Source: CAD feature listing. Evaluate the final solid. Frame: model axes, mm. A direction names the side the tool comes from. Coordinates: 2 decimals unless noted, no trailing zeros. Write each loop counter-clockwise with the first axis right and the second up, starting at its lowest first coordinate (ties: lowest second). Pieces come first, ordered by that corner, then holes. Notation, with made-up numbers: (22, 0.25) - (45, 0.25) arc R21 cw to (45, 16.25) - close; hole circle Ø5 at (50.25, 53). An arc over 180 degrees is marked (long way). One line per question, with ' | ' between items. Start each with the question number.
Q1. Draft query along Z for faces 1 (the face through (-4, 0, -482.6)), 2 (the face through (111, 0, 185.737)), 3 (the face through (136.525, 0, 405)). Return one class per face: +Z half, -Z half, draft (parallel to the pull), parting line (faces both ways), or undercut.
Q2. Line query: line 1 (Z direction, x = -250.5, y = 5.25); line 2 (X direction, y = 4.5, z = -330.2) (3 decimals); line 3 (X direction, y = -0.25, z = 275) (3 decimals). Output: solid intervals per line, ascending.
Q3. Contact query for flat-ended pins moving along their axis: P1, Ø4, axis at y = 1.5, z = 157, coming from the -X side (3 decimals); P2, Ø7.5, axis at x = 103.5, y = -1, coming from the +Z side. Output: stop coordinate, or through.
Q4. Cut plane A-A, the plane x = 116.5. Give the number of separate pieces and of enclosed holes in the cut face, plus the area to 3 significant figures.
Q5. Access query for faces 4 (the face through (-239, 0, 249.238)), 5 (the face through (111, 0, 58.738)), 6 (the face through (214, 0, 482.6)). Directions: +Z, -Z, +X, -X, +Y, -Y. A direction counts if a zero-diameter tool reaches every point of the face in a straight line with its end or side. Return the directions, or none.
Q6. Cut plane B-B, the plane z = -134.5. Return loops of the section in (x, y) (3 decimals), plus the area to 3 significant figures.
```python
from build123d import *

# Parameters (mm, degrees)
F1_DEPTH = 12.7
F2_R     = 6.35
F3_DEPTH = 25.4
F4_R     = 9.525
F5_DEPTH = 25.4
F6_W     = 50.8
F6_H     = 12.7
F7_DEPTH = 25.4


with BuildPart() as f1:
    # F0 (on Front) → F1 (new body, symmetric)
    with BuildSketch(Plane.XZ):
        Polygon((-288.925, -406.4), (-288.925, -482.6), (288.925, -482.6), (288.925, 482.6), (136.525, 482.6), (136.525, 325.4375), (-288.925, 325.4375), (-288.925, 249.2375), (-187.325, 249.2375), (-187.325, -406.4), align=None)
    extrude(amount=F1_DEPTH, both=True)

    # F2 (on face) → F3 (cut)
    with BuildSketch(Plane.XZ.offset(12.7)):
        with Locations((231.775, -330.2)):
            Circle(F2_R)
    extrude(amount=-F3_DEPTH, mode=Mode.SUBTRACT)

    # F4 (on face) → F5 (cut)
    with BuildSketch(Plane.XZ.offset(12.7)):
        with Locations((34.759605, -194.841525)):
            Circle(F4_R)
    extrude(amount=-F5_DEPTH, mode=Mode.SUBTRACT)

    # F6 (on face) → F7 (cut)
    with BuildSketch(Plane.XZ.offset(12.7)):
        with Locations((111.125, 306.3875)):
            Rectangle(F6_W, F6_H)
        with Locations((111.125, 280.9875)):
            Rectangle(F6_W, F6_H)
        with Locations((111.125, 255.5875)):
            Rectangle(F6_W, F6_H)
        with Locations((111.125, 230.1875)):
            Rectangle(F6_W, F6_H)
        with Locations((111.125, 204.7875)):
            Rectangle(F6_W, F6_H)
        with Locations((111.125, 179.3875)):
            Rectangle(F6_W, F6_H)
        with Locations((111.125, 153.9875)):
            Rectangle(F6_W, F6_H)
        with Locations((111.125, 128.5875)):
            Rectangle(F6_W, F6_H)
        with Locations((111.125, 103.1875)):
            Rectangle(F6_W, F6_H)
        with Locations((111.125, 77.7875)):
            Rectangle(F6_W, F6_H)
        with Locations((111.125, 52.3875)):
            Rectangle(F6_W, F6_H)
        with Locations((111.125, 26.9875)):
            Rectangle(F6_W, F6_H)
    extrude(amount=-F7_DEPTH, mode=Mode.SUBTRACT)


solid = f1.part
```
Reply:
1) face 1: -Z half | face 2: undercut | face 3: draft
2) line 1: z = -482.6 to -406.4, 249.24 to 325.44 | line 2: x = -187.325 to 225.425, 238.125 to 288.925 | line 3: x = -288.925 to 85.725, 136.525 to 288.925
3) P1: stops at x = -187.325 | P2: stops at z = 325.44
4) separate pieces: 13 | enclosed holes: 0 | area: 16,700 mm^2
5) face 4: -X, +Y, -Y | face 5: +Y, -Y | face 6: +Z, +X, -X, +Y, -Y
6) outline: (-187.325, -12.7) - (288.925, -12.7) - (288.925, 12.7) - (-187.325, 12.7) - close | area: 12,100 mm^2
